```python
from build123d import *

# Parameters (mm, degrees)
F0_W     = 300
F0_H     = 150
F0_R     = 7.65
F1_DEPTH = 3.5
F2_W     = 300
F2_H     = 150
F3_DEPTH = 15


with BuildPart() as f1:
    # F0 (on Front) → F1 (new body)
    with BuildSketch(Plane.XZ):
        with Locations((-180.280095, 78.015107)):
            Rectangle(F0_W, F0_H)
        with Locations((-292.164981, 29.736487)):
            Circle(F0_R, mode=Mode.SUBTRACT)
        with Locations((-267.164981, 29.736487)):
            Circle(F0_R, mode=Mode.SUBTRACT)
        with Locations((-242.164981, 29.736487)):
            Circle(F0_R, mode=Mode.SUBTRACT)
        with Locations((-217.164981, 29.736487)):
            Circle(F0_R, mode=Mode.SUBTRACT)
        with Locations((-192.164981, 29.736487)):
            Circle(F0_R, mode=Mode.SUBTRACT)
        with Locations((-292.164981, 54.736487)):
            Circle(F0_R, mode=Mode.SUBTRACT)
        with Locations((-267.164981, 54.736487)):
            Circle(F0_R, mode=Mode.SUBTRACT)
        with Locations((-242.164981, 54.736487)):
            Circle(F0_R, mode=Mode.SUBTRACT)
        with Locations((-217.164981, 54.736487)):
            Circle(F0_R, mode=Mode.SUBTRACT)
        with Locations((-192.164981, 54.736487)):
            Circle(F0_R, mode=Mode.SUBTRACT)
        with Locations((-167.164981, 29.736487)):
            Circle(F0_R, mode=Mode.SUBTRACT)
        with Locations((-142.164981, 29.736487)):
            Circle(F0_R, mode=Mode.SUBTRACT)
        with Locations((-117.164981, 29.736487)):
            Circle(F0_R, mode=Mode.SUBTRACT)
        with Locations((-92.164981, 29.736487)):
            Circle(F0_R, mode=Mode.SUBTRACT)
        with Locations((-67.164981, 29.736487)):
            Circle(F0_R, mode=Mode.SUBTRACT)
        with Locations((-167.164981, 54.736487)):
            Circle(F0_R, mode=Mode.SUBTRACT)
        with Locations((-142.164981, 54.736487)):
            Circle(F0_R, mode=Mode.SUBTRACT)
        with Locations((-117.164981, 54.736487)):
            Circle(F0_R, mode=Mode.SUBTRACT)
        with Locations((-92.164981, 54.736487)):
            Circle(F0_R, mode=Mode.SUBTRACT)
        with Locations((-67.164981, 54.736487)):
            Circle(F0_R, mode=Mode.SUBTRACT)
        with Locations((-292.164981, 79.736487)):
            Circle(F0_R, mode=Mode.SUBTRACT)
        with Locations((-267.164981, 79.736487)):
            Circle(F0_R, mode=Mode.SUBTRACT)
        with Locations((-292.164981, 104.736487)):
            Circle(F0_R, mode=Mode.SUBTRACT)
        with Locations((-267.164981, 104.736487)):
            Circle(F0_R, mode=Mode.SUBTRACT)
        with Locations((-242.164981, 79.736487)):
            Circle(F0_R, mode=Mode.SUBTRACT)
        with Locations((-217.164981, 79.736487)):
            Circle(F0_R, mode=Mode.SUBTRACT)
        with Locations((-192.164981, 79.736487)):
            Circle(F0_R, mode=Mode.SUBTRACT)
        with Locations((-242.164981, 104.736487)):
            Circle(F0_R, mode=Mode.SUBTRACT)
        with Locations((-217.164981, 104.736487)):
            Circle(F0_R, mode=Mode.SUBTRACT)
        with Locations((-192.164981, 104.736487)):
            Circle(F0_R, mode=Mode.SUBTRACT)
        with Locations((-292.164981, 129.736487)):
            Circle(F0_R, mode=Mode.SUBTRACT)
        with Locations((-267.164981, 129.736487)):
            Circle(F0_R, mode=Mode.SUBTRACT)
        with Locations((-242.164981, 129.736487)):
            Circle(F0_R, mode=Mode.SUBTRACT)
        with Locations((-217.164981, 129.736487)):
            Circle(F0_R, mode=Mode.SUBTRACT)
        with Locations((-192.164981, 129.736487)):
            Circle(F0_R, mode=Mode.SUBTRACT)
        with Locations((-167.164981, 79.736487)):
            Circle(F0_R, mode=Mode.SUBTRACT)
        with Locations((-142.164981, 79.736487)):
            Circle(F0_R, mode=Mode.SUBTRACT)
        with Locations((-117.164981, 79.736487)):
            Circle(F0_R, mode=Mode.SUBTRACT)
        with Locations((-167.164981, 104.736487)):
            Circle(F0_R, mode=Mode.SUBTRACT)
        with Locations((-142.164981, 104.736487)):
            Circle(F0_R, mode=Mode.SUBTRACT)
        with Locations((-117.164981, 104.736487)):
            Circle(F0_R, mode=Mode.SUBTRACT)
        with Locations((-92.164981, 79.736487)):
            Circle(F0_R, mode=Mode.SUBTRACT)
        with Locations((-67.164981, 79.736487)):
            Circle(F0_R, mode=Mode.SUBTRACT)
        with Locations((-92.164981, 104.736487)):
            Circle(F0_R, mode=Mode.SUBTRACT)
        with Locations((-67.164981, 104.736487)):
            Circle(F0_R, mode=Mode.SUBTRACT)
        with Locations((-167.164981, 129.736487)):
            Circle(F0_R, mode=Mode.SUBTRACT)
        with Locations((-142.164981, 129.736487)):
            Circle(F0_R, mode=Mode.SUBTRACT)
        with Locations((-117.164981, 129.736487)):
            Circle(F0_R, mode=Mode.SUBTRACT)
        with Locations((-92.164981, 129.736487)):
            Circle(F0_R, mode=Mode.SUBTRACT)
        with Locations((-67.164981, 129.736487)):
            Circle(F0_R, mode=Mode.SUBTRACT)
    extrude(amount=F1_DEPTH)

    # F2 (on Front) → F3 (join)
    with BuildSketch(Plane.XZ):
        with Locations((-180.280095, 78.015107)):
            Rectangle(F2_W, F2_H)
    extrude(amount=-F3_DEPTH)


solid = f1.part
```
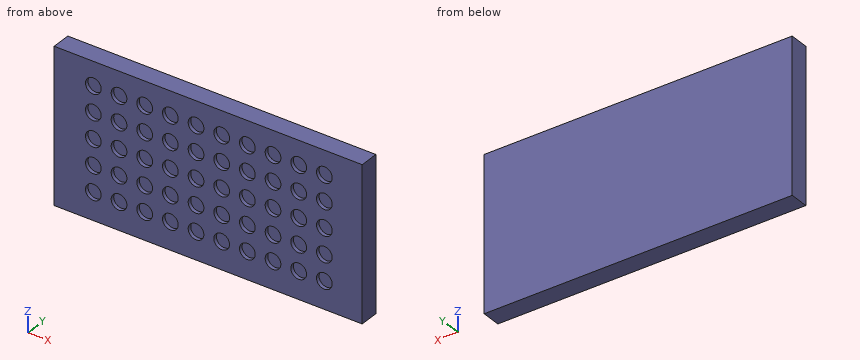
Model file for the job. Use its own axes, mm. Coordinates: 2 decimals unless noted, no trailing zeros. Write each loop counter-clockwise with the first axis right and the second up, starting at its lowest first coordinate (ties: lowest second). Pieces come first, ordered by that corner, then holes. Notation, with made-up numbers: (5, 41) - (13, 41) arc R22 cw to (13, 68) - close; hole circle Ø7 at (42.25, 59). An arc over 180 degrees is marked (long way). One line per question, with ' | ' between items. Start each with the question number.
Q1. Drill centre lines: line 1 (Z direction, x = -266.5, y = -1.25); line 2 (Z direction, x = -218.5, y = -0.5); line 3 (Y direction, x = -70, z = 52). Where is each one in solid material? Low to high. Write a range as [from, to].
Q2. Pin check, flat tip, straight feed: pin 1 (7.5 mm diameter, centred on x = -265.5, z = 132, fed in from -Y). Stop position of the tip, or through.
Q3. Cut at B-B, the plane x = -67.5. List the corners of the cut face in (y, z), then the cut area to 3 significant figures.
Q4. Cut at A-A, the plane x = -195. List the corners of the cut face in (y, z), then the cut area to 3 significant figures.
Answer below:
1) line 1: [3.02, 22.12], [37.36, 47.12], [62.36, 72.12], [87.36, 97.12], [112.36, 122.12], [137.36, 153.02] | line 2: [3.02, 22.2], [37.27, 47.2], [62.27, 72.2], [87.27, 97.2], [112.27, 122.2], [137.27, 153.02] | line 3: [0, 15]
2) pin 1: y = 0
3) outline: (-3.5, 3.02) - (15, 3.02) - (15, 153.02) - (-3.5, 153.02) - (-3.5, 137.38) - (0, 137.38) - (0, 122.09) - (-3.5, 122.09) - (-3.5, 112.38) - (0, 112.38) - (0, 97.09) - (-3.5, 97.09) - (-3.5, 87.38) - (0, 87.38) - (0, 72.09) - (-3.5, 72.09) - (-3.5, 62.38) - (0, 62.38) - (0, 47.09) - (-3.5, 47.09) - (-3.5, 37.38) - (0, 37.38) - (0, 22.09) - (-3.5, 22.09) - close | area: 2,510 mm^2
4) outline: (-3.5, 3.02) - (15, 3.02) - (15, 153.02) - (-3.5, 153.02) - (-3.5, 136.84) - (0, 136.84) - (0, 122.63) - (-3.5, 122.63) - (-3.5, 111.84) - (0, 111.84) - (0, 97.63) - (-3.5, 97.63) - (-3.5, 86.84) - (0, 86.84) - (0, 72.63) - (-3.5, 72.63) - (-3.5, 61.84) - (0, 61.84) - (0, 47.63) - (-3.5, 47.63) - (-3.5, 36.84) - (0, 36.84) - (0, 22.63) - (-3.5, 22.63) - close | area: 2,530 mm^2
